```python
from build123d import *

# Parameters (mm, degrees)
SKETCH1_R           = 1.6
BOSS_EXTRUDE1_DEPTH = 4
CUT_EXTRUDE1_DEPTH  = 2
FILLET2_R           = 30
CUT_EXTRUDE5_DEPTH  = 52.039200621
SKETCH7_W           = 35
SKETCH7_H           = 20
CUT_EXTRUDE6_DEPTH  = 52.039200621


with BuildPart() as part:
    # Sketch1 → Boss-Extrude1 (new body)
    with BuildSketch(Plane(origin=(0, 0, 0), x_dir=(1, 0, 0), z_dir=(0, 1, 0))):
        Polygon((-12.5, 35), (12.5, 35), (23.334523779, 36.062445841), (36.062445841, 23.334523779), (35, 12.5), (35, -12.5), (36.062445841, -23.334523779), (23.334523779, -36.062445841), (12.5, -35), (-12.5, -35), (-23.334523779, -36.062445841), (-36.06244584, -23.334523779), (-35, -12.5), (-35, 12.5), (-36.062445841, 23.334523779), (-23.334523779, 36.062445841), align=None)
        with Locations(Location((22.627416998, 31.112698372, 0), (0, 0, 270))):
            Circle(SKETCH1_R, mode=Mode.SUBTRACT)
        with Locations(Location((31.112698372, 22.627416998, 0), (0, 0, 270))):
            Circle(SKETCH1_R, mode=Mode.SUBTRACT)
        with Locations(Location((22.627416998, -31.112698372, 0), (0, 0, 270))):
            Circle(SKETCH1_R, mode=Mode.SUBTRACT)
        with Locations(Location((31.112698372, -22.627416998, 0), (0, 0, 270))):
            Circle(SKETCH1_R, mode=Mode.SUBTRACT)
        with Locations(Location((-31.112698372, -22.627416998, 0), (0, 0, 270))):
            Circle(SKETCH1_R, mode=Mode.SUBTRACT)
        with Locations(Location((-22.627416998, -31.112698372, 0), (0, 0, 270))):
            Circle(SKETCH1_R, mode=Mode.SUBTRACT)
        with Locations(Location((-22.627416998, 31.112698372, 0), (0, 0, 270))):
            Circle(SKETCH1_R, mode=Mode.SUBTRACT)
        with Locations(Location((-31.112698372, 22.627416998, 0), (0, 0, 270))):
            Circle(SKETCH1_R, mode=Mode.SUBTRACT)
    extrude(amount=BOSS_EXTRUDE1_DEPTH)

    # Sketch2 → Cut-Extrude1 (cut)
    with BuildSketch(Plane(origin=(0, 4, 0), x_dir=(1, 0, 0), z_dir=(0, 1, 0))):
        Polygon((-17.669047558, 29), (17.669047558, 29), (29, 17.669047558), (29, -17.669047558), (17.669047558, -29), (-17.669047558, -29), (-29, -17.669047558), (-29, 17.669047558), align=None)
    extrude(amount=-CUT_EXTRUDE1_DEPTH, mode=Mode.SUBTRACT)

    # Fillet2
    # the kernel refuses this fillet: 30 mm, written as the material it adds along each edge
    with BuildSketch(Plane(origin=(-12.5, 0, -35), x_dir=(1, 0, 0), z_dir=(0, 1, 0))) as fillet2_piece_1:
        with BuildLine():
            CenterArc((FILLET2_R * 0.0489132680017, FILLET2_R), FILLET2_R, 264.399415997, 5.600584003)
            Line((-FILLET2_R * 0.0486797758843, FILLET2_R * 0.00477359471069), (0, 0))
            Line((0, 0), (FILLET2_R * 0.0489132680017, 0))
        make_face()
    extrude(amount=4)
    with BuildSketch(Plane(origin=(12.5, 0, -35), x_dir=(-1, 0, 0), z_dir=(0, 1, 0)), Plane(origin=(35, 0, -12.5), x_dir=(0.09759304388595028, 0, -0.9952264052893065), z_dir=(0, 1, 0)), Plane(origin=(35, 0, 12.5), x_dir=(0, 0, -1), z_dir=(0, 1, 0)), Plane(origin=(12.5, 0, 35), x_dir=(0.9952264052893073, 0, 0.09759304388594116), z_dir=(0, 1, 0)), Plane(origin=(-12.5, 0, 35), x_dir=(1, 0, 0), z_dir=(0, 1, 0)), Plane(origin=(-35, 0, 12.5), x_dir=(-0.09759304388594536, 0, 0.995226405289307), z_dir=(0, 1, 0)), Plane(origin=(-35, 0, -12.5), x_dir=(0, 0, 1), z_dir=(0, 1, 0))) as fillet2_piece_2:
        with BuildLine():
            CenterArc((FILLET2_R * 0.048913268002, -FILLET2_R), FILLET2_R, 90, 5.600584003)
            Line((-FILLET2_R * 0.0486797758846, -FILLET2_R * 0.00477359471075), (0, 0))
            Line((0, 0), (FILLET2_R * 0.048913268002, 0))
        make_face()
    extrude(amount=4)

    # Sketch6 → Cut-Extrude5 (cut, through all)
    with BuildSketch(Plane(origin=(0, 2, 0), x_dir=(1, 0, 0), z_dir=(0, 1, 0))):
        with BuildLine():
            Line((-1.5, 19.7), (-1.5, 18.3))
            ThreePointArc((-1.5, 18.3), (-1.734314575, 17.734314575), (-2.3, 17.5))
            Line((-2.3, 17.5), (-6.7, 17.5))
            ThreePointArc((-6.7, 17.5), (-7.265685425, 17.734314575), (-7.5, 18.3))
            Line((-7.5, 18.3), (-7.5, 26.7))
            ThreePointArc((-7.5, 26.7), (-7.265685425, 27.265685425), (-6.7, 27.5))
            Line((-6.7, 27.5), (6.7, 27.5))
            ThreePointArc((6.7, 27.5), (7.265685425, 27.265685425), (7.5, 26.7))
            Line((7.5, 26.7), (7.5, 18.3))
            ThreePointArc((7.5, 18.3), (7.265685425, 17.734314575), (6.7, 17.5))
            Line((6.7, 17.5), (2.3, 17.5))
            ThreePointArc((2.3, 17.5), (1.734314575, 17.734314575), (1.5, 18.3))
            Line((1.5, 18.3), (1.5, 19.7))
            ThreePointArc((1.5, 19.7), (1.734314575, 20.265685425), (2.3, 20.5))
            Line((2.3, 20.5), (4.2, 20.5))
            ThreePointArc((4.2, 20.5), (4.765685425, 20.734314575), (5, 21.3))
            Line((5, 21.3), (5, 23.7))
            ThreePointArc((5, 23.7), (4.765685425, 24.265685425), (4.2, 24.5))
            Line((4.2, 24.5), (-4.2, 24.5))
            ThreePointArc((-4.2, 24.5), (-4.765685425, 24.265685425), (-5, 23.7))
            Line((-5, 23.7), (-5, 21.3))
            ThreePointArc((-5, 21.3), (-4.765685425, 20.734314575), (-4.2, 20.5))
            Line((-4.2, 20.5), (-2.3, 20.5))
            ThreePointArc((-2.3, 20.5), (-1.734314575, 20.265685425), (-1.5, 19.7))
        make_face()
        with BuildLine():
            Line((-2.3, -17.5), (-6.7, -17.5))
            ThreePointArc((-6.7, -17.5), (-7.265685425, -17.734314575), (-7.5, -18.3))
            Line((-7.5, -18.3), (-7.5, -26.7))
            ThreePointArc((-7.5, -26.7), (-7.265685425, -27.265685425), (-6.7, -27.5))
            Line((-6.7, -27.5), (6.7, -27.5))
            ThreePointArc((6.7, -27.5), (7.265685425, -27.265685425), (7.5, -26.7))
            Line((7.5, -26.7), (7.5, -18.3))
            ThreePointArc((7.5, -18.3), (7.265685425, -17.734314575), (6.7, -17.5))
            Line((6.7, -17.5), (2.3, -17.5))
            ThreePointArc((2.3, -17.5), (1.734314575, -17.734314575), (1.5, -18.3))
            Line((1.5, -18.3), (1.5, -19.7))
            ThreePointArc((1.5, -19.7), (1.734314575, -20.265685425), (2.3, -20.5))
            Line((2.3, -20.5), (4.2, -20.5))
            ThreePointArc((4.2, -20.5), (4.765685425, -20.734314575), (5, -21.3))
            Line((5, -21.3), (5, -23.7))
            ThreePointArc((5, -23.7), (4.765685425, -24.265685425), (4.2, -24.5))
            Line((4.2, -24.5), (-4.2, -24.5))
            ThreePointArc((-4.2, -24.5), (-4.765685425, -24.265685425), (-5, -23.7))
            Line((-5, -23.7), (-5, -21.3))
            ThreePointArc((-5, -21.3), (-4.765685425, -20.734314575), (-4.2, -20.5))
            Line((-4.2, -20.5), (-2.3, -20.5))
            ThreePointArc((-2.3, -20.5), (-1.734314575, -20.265685425), (-1.5, -19.7))
            Line((-1.5, -19.7), (-1.5, -18.3))
            ThreePointArc((-1.5, -18.3), (-1.734314575, -17.734314575), (-2.3, -17.5))
        make_face()
    extrude(amount=-CUT_EXTRUDE5_DEPTH, mode=Mode.SUBTRACT)

    # Sketch7 → Cut-Extrude6 (cut, through all)
    with BuildSketch(Plane(origin=(0, 2, 0), x_dir=(1, 0, 0), z_dir=(0, 1, 0))):
        Rectangle(SKETCH7_W, SKETCH7_H)
    extrude(amount=-CUT_EXTRUDE6_DEPTH, mode=Mode.SUBTRACT)


solid = part.part
```
Build history of the part. All positions in model axes, mm. A direction names the side the tool comes from. Round coordinates to 2 decimals unless told otherwise and drop trailing zeros. Loops run counter-clockwise (first coordinate to the right, second up) from the corner with the lowest first, then second, coordinate; pieces in that order, holes last. Notation, with made-up numbers: M -28.75,0.5 L -21.75,0.5 A23 cw -21.75,28.5 Z; hole C 58.5,-11.5 d4. An arc over 180 degrees is marked long. Answer as CSV lines item,"result".
1. Cut at C-C on z = -22.5. Write the cut outline in (x, y), then the cut area to 3 significant figures.
Resolved:
outline,"M -35.98,0 L -32.71,0 L -32.71,4 L -35.98,4 Z; M -29.52,0 L -7.5,0 L -7.5,2 L -24.17,2 L -24.17,4 L -29.52,4 Z; M -5,0 L 5,0 L 5,2 L -5,2 Z; M 7.5,0 L 29.52,0 L 29.52,4 L 24.17,4 L 24.17,2 L 7.5,2 Z; M 32.71,0 L 35.98,0 L 35.98,4 L 32.71,4 Z"
area,"156 mm²"
2. Cut at D-D on x = 18.5. Write the cut outline in (y, z).
Resolved:
outline,"M 0,-35.59 L 4,-35.59 L 4,-28.17 L 2,-28.17 L 2,28.17 L 4,28.17 L 4,35.59 L 0,35.59 Z"
3. 3-axis set-ups, long thin cutter, end or side, ignore diameter. For faces 1 (the flat face through (-35.61, 1.97, 18.71)), 2 (the flat face through (-18.6, 2, 35.6)), 3 (the flat face through (-5, 1, -23)): which of +Z, -Z, +X, -X, +Y, -Y reach the whole face in a straight line?
Resolved:
face 1,"-X, +Y, -Y"
face 2,"+Z, +Y, -Y"
face 3,"+Y, -Y"
4. Two-plate mould, pull along Z, no slides. Class faces 4 (the cylindrical face through (22.01, 1.97, 32.59)), 5 (the flat face through (-1, 0, 17)), 6 (the flat face through (29.788, 1.972, 29.609)), 7 (the cylindrical face through (-22.56, 1.97, -32.71)): released by +Z, released by -Z, zero draft, split by the parting line, or undercut.
Resolved:
face 4,"undercut"
face 5,"zero draft"
face 6,"released by +Z"
face 7,"undercut"
5. Wall check: probe 1 along Z at (x, y) = (-6, 1); probe 2 along Z at (x, y) = (12, 0.3); probe 3 along X at (y, z) = (1.55, 18). Give the ranges that are in metal, low to high. Write a range as [from, to].
Resolved:
probe 1,"z = [-35, -27.5], [-17.5, -10], [10, 17.5], [27.5, 35]"
probe 2,"z = [-35.02, -10], [10, 35.02]"
probe 3,"x = [-35.54, -7.44], [-1.56, 1.56], [7.44, 35.54]"
6. Flat gauge pins, fed straight in: P1, Ø1, axis at x = 27.5, y = 0.5, coming from the +Z side; P2, Ø2, axis at x = 2, y = 2.5, coming from the +Z side; P3, Ø12, axis at x = 16.5, z = 1.5, coming from the +Y side; P4, Ø4, axis at x = -22.63, z = 31.11, coming from the +Y side. Where does each tip first touch, or does it go through?
Resolved:
P1,"stops at z = 32.4"
P2,"stops at z = 35"
P3,"stops at y = 2"
P4,"stops at y = 4"
7. Cut at B-B on z = -0.5. Write the cut outline in (x, y).
Resolved:
outline,"M -35,0 L -17.5,0 L -17.5,2 L -29,2 L -29,4 L -35,4 Z; M 17.5,0 L 35,0 L 35,4 L 29,4 L 29,2 L 17.5,2 Z"
8. Cut at A-A on x = -10. Write the cut outline in (y, z), then the cut area to 3 significant figures.
Resolved:
outline,"M 0,-35 L 4,-35 L 4,-29 L 2,-29 L 2,-10 L 0,-10 Z; M 0,10 L 2,10 L 2,29 L 4,29 L 4,35 L 0,35 Z"
area,"124 mm²"
